from build123d import *

# Parameters (mm, degrees)
F0_R     = 1.5875
F1_DEPTH = 25.4


# Not quite as in the source:
# - ends of sketch curves that miss each other by under 0.0002 mm in the source are joined


with BuildPart() as f1:
    # F0 (on Front) → F1 (new body)
    with BuildSketch(Plane.XZ):
        with BuildLine():
            ThreePointArc((1.5875, 0), (-1.1225320151, -1.1225320151), (0, 1.5875))
            Line((0, 1.5875), (0, 9.525))
            ThreePointArc((0, 9.525), (-6.5322234356, 6.9322205668), (-9.5082023407, 0.5654319132))
            ThreePointArc((-9.5082023407, 0.5654319132), (-6.9322205668, -6.5322234356), (0, -9.525))
            Line((0, -9.525), (0.6773435479, -9.500885786))
            ThreePointArc((0.6773435479, -9.500885786), (6.9705567315, -6.4912990883), (9.525, 0))
            Line((9.525, 0), (1.5875, 0))
        make_face()
        with BuildLine():
            ThreePointArc((-9.5082023407, 0.5654319132), (-6.5322234356, 6.9322205668), (0, 9.525))
            Line((0, 9.525), (0, 47.625))
            ThreePointArc((0, 47.625), (-10.5003255158, 51.59375), (-15.7504882737, 61.515625))
            Line((-15.7504882737, 61.515625), (-9.5082023407, 0.5654319132))
        make_face()
        with BuildLine():
            Line((0, 47.625), (0, 9.525))
            ThreePointArc((0, 9.525), (0.3388863295, 9.5189695375), (0.6773435479, 9.500885786))
            Line((0.6773435479, 9.500885786), (10.4519953809, 9.152896871))
            Line((10.4519953809, 9.152896871), (15.7942028036, 61.9003804205))
            ThreePointArc((15.7942028036, 61.9003804205), (10.644756084, 51.722700101), (0, 47.625))
        make_face()
        with BuildLine():
            Line((10.4519953809, 9.152896871), (9.525, 0))
            Line((9.525, 0), (36.5125, 0))
            ThreePointArc((36.5125, 0), (38.9380895153, 5.7116327839), (44.7324052746, 7.9324746146))
            Line((44.7324052746, 7.9324746146), (10.4519953809, 9.152896871))
        make_face()
        with BuildLine():
            Line((36.5125, 0), (9.525, 0))
            ThreePointArc((9.525, 0), (6.9705567315, -6.4912990883), (0.6773435479, -9.500885786))
            Line((0.6773435479, -9.500885786), (44.7324052746, -7.9324746146))
            ThreePointArc((44.7324052746, -7.9324746146), (38.9380895153, -5.7116327839), (36.5125, 0))
        make_face()
        with BuildLine():
            ThreePointArc((0.6773435479, 9.500885786), (6.9705567315, 6.4912990883), (9.525, 0))
            Line((9.525, 0), (10.4519953809, 9.152896871))
            Line((10.4519953809, 9.152896871), (0.6773435479, 9.500885786))
        make_face()
        with BuildLine():
            ThreePointArc((-15.7504882737, 61.515625), (-10.5003255158, 51.59375), (0, 47.625))
            Line((0, 47.625), (0, 61.9125))
            ThreePointArc((0, 61.9125), (-1.5875, 63.5), (0, 65.0875))
            Line((0, 65.0875), (0, 79.375))
            ThreePointArc((0, 79.375), (-10.5003255158, 75.40625), (-15.7504882737, 65.484375))
            ThreePointArc((-15.7504882737, 65.484375), (-15.875, 63.5), (-15.7504882737, 61.515625))
        make_face()
        with BuildLine():
            ThreePointArc((0, 79.375), (10.5154665352, 75.3928797415), (15.7554871092, 65.444286746))
            Line((15.7554871092, 65.444286746), (9.4502929642, 115.490625))
            ThreePointArc((9.4502929642, 115.490625), (9.5063048942, 114.896483242), (9.525, 114.3))
            ThreePointArc((9.525, 114.3), (6.7351920908, 107.5648079092), (0, 104.775))
            Line((0, 104.775), (0, 79.375))
        make_face()
        with BuildLine():
            Line((0, 61.9125), (0, 47.625))
            ThreePointArc((0, 47.625), (10.644756084, 51.722700101), (15.7942028036, 61.9003804205))
            ThreePointArc((15.7942028036, 61.9003804205), (15.8547878338, 62.6991705884), (15.875, 63.5))
            ThreePointArc((15.875, 63.5), (15.8450936075, 64.4739782187), (15.7554871092, 65.444286746))
            ThreePointArc((15.7554871092, 65.444286746), (10.5154665352, 75.3928797415), (0, 79.375))
            Line((0, 79.375), (0, 65.0875))
            ThreePointArc((0, 65.0875), (1.1225320151, 64.6225320151), (1.5875, 63.5))
            ThreePointArc((1.5875, 63.5), (1.1225320151, 62.3774679849), (0, 61.9125))
        make_face()
        with BuildLine():
            ThreePointArc((44.7324052746, 7.9324746146), (38.9380895153, 5.7116327839), (36.5125, 0))
            ThreePointArc((36.5125, 0), (38.9380895153, -5.7116327839), (44.7324052746, -7.9324746146))
            ThreePointArc((44.7324052746, -7.9324746146), (50.1616327839, -5.5119104847), (52.3875, 0))
            ThreePointArc((52.3875, 0), (50.1616327839, 5.5119104847), (44.7324052746, 7.9324746146))
        make_face()
        with BuildLine():
            ThreePointArc((46.0375, 0), (44.45, -1.5875), (42.8625, 0))
            ThreePointArc((42.8625, 0), (44.45, 1.5875), (46.0375, 0))
        make_face(mode=Mode.SUBTRACT)
        with BuildLine():
            ThreePointArc((0, -9.525), (0.3388863295, -9.5189695375), (0.6773435479, -9.500885786))
            Line((0.6773435479, -9.500885786), (0, -9.525))
        make_face()
        with BuildLine():
            Line((-9.4502929642, 115.490625), (-15.7504882737, 65.484375))
            ThreePointArc((-15.7504882737, 65.484375), (-10.5003255158, 75.40625), (0, 79.375))
            Line((0, 79.375), (0, 104.775))
            ThreePointArc((0, 104.775), (-7.14375, 107.9998046905), (-9.4502929642, 115.490625))
        make_face()
        with Locations((-2.919731196, 102.79443115)):
            Circle(F0_R, mode=Mode.SUBTRACT)
        with BuildLine():
            ThreePointArc((9.4502929642, 115.490625), (0, 123.825), (-9.4502929642, 115.490625))
            ThreePointArc((-9.4502929642, 115.490625), (-7.14375, 107.9998046905), (0, 104.775))
            ThreePointArc((0, 104.775), (6.7351920908, 107.5648079092), (9.525, 114.3))
            ThreePointArc((9.525, 114.3), (9.5063048942, 114.896483242), (9.4502929642, 115.490625))
        make_face()
        with BuildLine():
            ThreePointArc((1.5875, 114.3), (1.1225320151, 113.1774679849), (0, 112.7125))
            ThreePointArc((0, 112.7125), (-1.1225320151, 115.4225320151), (1.5875, 114.3))
        make_face(mode=Mode.SUBTRACT)
        with BuildLine():
            Line((0, 9.525), (0, 1.5875))
            ThreePointArc((0, 1.5875), (1.1225320151, 1.1225320151), (1.5875, 0))
            Line((1.5875, 0), (9.525, 0))
            ThreePointArc((9.525, 0), (6.9705567315, 6.4912990883), (0.6773435479, 9.500885786))
            Line((0.6773435479, 9.500885786), (0, 9.525))
        make_face()
    extrude(amount=F1_DEPTH)


solid = f1.part
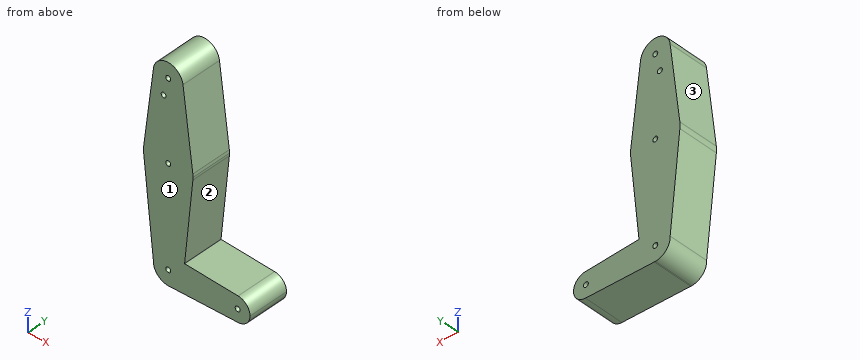
Part model, mm, in its own coordinate system. Face numbers are marked on the shaded views. Give positions to 0.01 mm unless a question says otherwise; leave off trailing zeros. Order: outer loops, then holes, each group sorted by start corner. A loop starts at its lowest first (then second) coordinate and runs counter-clockwise, first axis right, second up. Notation, with made-up numbers: (-33, 4.25) - (21, 4.25) arc R32 ccw to (21, 33.25) - close; hole circle Ø9 at (57, -6). An arc over 180 degrees is marked (long way). Use a Markdown table: item, result.
1) Saw through at B-B on z = 29.5. List the corners of the cut face in (x, y).
Checked values:
| item | result |
|---|---|
| outline | (-12.47, -25.4) - (12.51, -25.4) - (12.51, 0) - (-12.47, 0) - close |
2) Flat gauge pins, fed straight in: P1, Ø3, axis at x = 44.45, z = 0, coming from the +Y side; P2, Ø3, axis at x = 38.5, y = -22.5, coming from the +Z side; P3, Ø12, axis at y = -13.5, z = 84, coming from the +X side; P4, Ø5, axis at x = 31.5, y = -21, coming from the -Z side. Where does each tip first touch, or does it go through?
Checked values:
| item | result |
|---|---|
| P1 | through |
| P2 | z = 8.21 |
| P3 | x = 14.17 |
| P4 | z = -8.49 |
3) Probe L1, parallel to X at y = -8.5, z = 0 (1 decimal); L2, parallel to X at y = -11, z = 65.5; L3, parallel to X at y = -13, z = 114.3. List the from-to ranges inside material, lowest first. Write a range as from..to.
Checked values:
| item | result |
|---|---|
| L1 | -9.5..-1.6, 1.6..42.9, 46..52.4 |
| L2 | -15.75..15.75 |
| L3 | -9.6..-1.59, 1.59..9.6 |
4) Two-plate mould, pull along Z, no slides. Class the marked faces 1, 2 and 3: +Z half, -Z half, draft (parallel to the pull), parting line (faces both ways), or undercut.
Checked values:
| item | result |
|---|---|
| face 1 | draft |
| face 2 | undercut |
| face 3 | +Z half |
5) Saw through at C-C on x = 19. List the corners of the cut face in (y, z), plus the area to 3 significant figures.
Checked values:
| item | result |
|---|---|
| outline | (-25.4, -8.85) - (0, -8.85) - (0, 8.85) - (-25.4, 8.85) - close |
| area | 450 mm² |
6) Saw through at A-A on y = -6.25. Count the separate pieces of the cut face and the enclosed holes in it, plus the area to 3 significant figures.
Checked values:
| item | result |
|---|---|
| separate pieces | 1 |
| enclosed holes | 6 |
| area | 3,870 mm² |
